from build123d import *

# Parameters (mm, degrees)
F0_R           = 25
F0_R_2         = 10
F1_DEPTH       = 130
F2_R           = 15
F3_DEPTH       = 20
F4_W           = 74.8539417982
F4_H           = 49.5208390057
F5_DEPTH       = 20.001
F5_DEPTH_BACK  = 130.001
F7_D           = 3.3
F7_DEPTH       = 6
F7_CSINK_D     = 6.72
F7_CSINK_ANGLE = 90
F7_TIP         = 0.9914200214


with BuildPart() as f1:
    # F0 (on Top) → F1 (new body)
    with BuildSketch(Plane.XY):
        Circle(F0_R)
        Circle(F0_R_2, mode=Mode.SUBTRACT)
        Circle(F0_R_2)
    extrude(amount=-F1_DEPTH)

    # F2
    f2_edges = [f1.edges().sort_by_distance(p)[0] for p in [
        (-25, 0, 0),
    ]]
    fillet(f2_edges, radius=F2_R)

    # F0 (on Top) → F3 (join)
    with BuildSketch(Plane.XY):
        Circle(F0_R_2)
    extrude(amount=F3_DEPTH)

    # F4 (on Top) → F5 (cut, two sides)
    with BuildSketch(Plane.XY) as f5_sk:
        with Locations((37.4269708991, -24.7604195029)):
            Rectangle(F4_W, F4_H)
    extrude(amount=F5_DEPTH, mode=Mode.SUBTRACT)
    extrude(f5_sk.sketch, amount=-F5_DEPTH_BACK, mode=Mode.SUBTRACT)

    # F7
    with Locations(Plane.XY.offset(20)):
        with Locations((0, 4)):
            CounterSinkHole(F7_D / 2, F7_CSINK_D / 2, depth=F7_DEPTH, counter_sink_angle=F7_CSINK_ANGLE)
            with Locations((0, 0, -(F7_DEPTH + F7_TIP / 2))):  # 118° drill point
                Cone(0, F7_D / 2, F7_TIP, mode=Mode.SUBTRACT)


solid = f1.part
For this review, take the finished solid that the model builds, in its own axes (mm). A direction names the side the tool comes from. Give positions to 0.01 mm unless a question says otherwise; leave off trailing zeros. Order: outer loops, then holes, each group sorted by start corner. A loop starts at its lowest first (then second) coordinate and runs counter-clockwise, first axis right, second up. Notation, with made-up numbers: (29.5, 75.5) - (74.5, 75.5) arc R7 cw to (74.5, 80.5) - close; hole circle Ø8 at (-34.5, 50). An arc over 180 degrees is marked (long way). Answer as a JSON object with one key per item and string values. Group by question number.
Item 1: Clearance check with flat-ended pins moving along their axes: pin 1 Ø3 at (x, z) = (-11, -101) entering from +Y; pin 2 Ø12.5 at (y, z) = (-9.5, -25) entering from +X; pin 3 Ø4 at (y, z) = (10, -51.5) entering from +X. State where each tip first meets the part, or that it passes through.
Item 2: Machinability: for faces 4 (the flat face through (-0.14, 0.14, 20)), 5 (the flat face through (0, -13, -56)), which of the approach directions +Z, -Z, +X, -X, +Y, -Y give a long, thin tool a straight path to every point of the face, cutting with its end or side? Answer none if there is none.
Item 3: Draft analysis for pull direction Y (two halves, no side actions). For faces 1 (the cylindrical face through (0.4, 2.4, 16.1)), 2 (the cylindrical face through (-6.834, 7.3, 9.86)), 3 (the flat face through (-0.3, 0.4, -130)), state which applies: pulls with the +Y half, pulls with the -Y half, needs draft (parallel to the pull), parting line crosses it, or undercut.
Item 4: Wall thickness on line 1 along X through (y, z) = (4, 16.8); line 2 along Z through (x, y) = (-19, 3.5); line 3 along X through (y, z) = (-8, -4.5): over which ranges is each line inside the solid? List them lowest first.
Item 5: Take a section at B-B on z = -95. Give the boundary of the cut face in (x, y).
Item 6: Take a section at A-A on z = 7. Give the boundary of the cut face in (x, y).
Reported:
{
 "1": {"pin 1": "y = 23.12", "pin 2": "x = 0", "pin 3": "x = 23.69"},
 "2": {"face 4": "+Z, +X, -X, +Y, -Y", "face 5": "+Z, -Z, +X, -Y"},
 "3": {"face 1": "undercut", "face 2": "parting line crosses it", "face 3": "needs draft"},
 "4": {"line 1": "-9.17 to -1.65, 1.65 to 9.17", "line 2": "-130 to -3.25", "line 3": "-19.1 to 0"},
 "5": {"outline": "(0, -25) - (0, 0) - (25, 0) arc R25 ccw (long way) to start"},
 "6": {"outline": "(0, -10) - (0, 0) - (10, 0) arc R10 ccw (long way) to start"}
}
